For this review, take the finished solid that the model builds, in its own axes (mm). A direction names the side the tool comes from. Coordinates: 2 decimals unless noted, no trailing zeros. Write each loop counter-clockwise with the first axis right and the second up, starting at its lowest first coordinate (ties: lowest second). Pieces come first, ordered by that corner, then holes. Notation, with made-up numbers: M 66,6.5 L 121,6.5 A15 ccw 121,13.5 Z; hole C -36.75,25.5 d10. An arc over 180 degrees is marked long. Return JSON: item names as keys, results as strings.
```python
from build123d import *

# Parameters (mm, degrees)
ESQUISSE1_W             = 5
ESQUISSE1_H             = 83
BOSS_EXTRU_1_DEPTH      = 18
TROU_TARAUD_M4_D        = 3.3
ESQUISSE4_W             = 5
ESQUISSE4_H             = 63
ENL_V_MAT_EXTRU_1_DEPTH = 10


with BuildPart() as part:
    # Esquisse1 → Boss.-Extru.1 (new body)
    with BuildSketch(Plane.XY):
        with Locations((0, 36.5)):
            Rectangle(ESQUISSE1_W, ESQUISSE1_H)
    extrude(amount=-BOSS_EXTRU_1_DEPTH)

    # Trou taraudé M4 (through all)
    with Locations(Plane.XY):
        with Locations((0, 0), (0, 36.5), (0, 73)):
            Hole(TROU_TARAUD_M4_D / 2)

    # Esquisse4 → Enlèv. mat.-Extru.1 (cut)
    with BuildSketch(Plane.XY):
        with Locations((0, 36.5)):
            Rectangle(ESQUISSE4_W, ESQUISSE4_H)
    extrude(amount=-ENL_V_MAT_EXTRU_1_DEPTH, mode=Mode.SUBTRACT)


solid = part.part
```
1. Wall thickness on L1, parallel to Y at x = 0, z = -14.5; L2, parallel to Y at x = 0, z = -7.25; L3, parallel to X at y = 73, z = -3.5: over which ranges is each line inside the solid? List them lowest first. Write a range as from..to.
Checks:
{"L1": "-5..-1.65, 1.65..34.85, 38.15..71.35, 74.65..78", "L2": "-5..-1.65, 1.65..5, 68..71.35, 74.65..78", "L3": "-2.5..-1.65, 1.65..2.5"}
2. We need section A-A (y = 0). State the section outline as (x, z) points.
Checks:
{"outline": "M -2.5,-18 L -1.65,-18 L -1.65,0 L -2.5,0 Z; M 1.65,-18 L 2.5,-18 L 2.5,0 L 1.65,0 Z"}
3. For faces 1 (the face through (2, 37, -10)), 2 (the face through (0, -5, -9)), list the 3-axis set-ups (+Z, -Z, +X, -X, +Y, -Y) from which the entire face can be reached by the end or side of a thin tool; tool diameter is ignored.
Checks:
{"face 1": "+Z, +X, -X", "face 2": "+Z, -Z, +X, -X, -Y"}
4. We need section D-D (y = 36.5). State the section outline as (x, z) points, plus the area to 3 significant figures.
Checks:
{"outline": "M -2.5,-18 L -1.65,-18 L -1.65,-10 L -2.5,-10 Z; M 1.65,-18 L 2.5,-18 L 2.5,-10 L 1.65,-10 Z", "area": "13.6 mm2"}
5. We need section C-C (z = -16). State the section outline as (x, y) points, plus the area to 3 significant figures.
Checks:
{"outline": "M -2.5,-5 L 2.5,-5 L 2.5,78 L -2.5,78 Z; hole C 0,0 d3.3; hole C 0,36.5 d3.3; hole C 0,73 d3.3", "area": "389 mm2"}
6. We need section B-B (x = 0). State the section outline as (y, z) points, plus the area to 3 significant figures.
Checks:
{"outline": "M -5,-18 L -1.65,-18 L -1.65,0 L -5,0 Z; M 1.65,-18 L 34.85,-18 L 34.85,-10 L 5,-10 L 5,0 L 1.65,0 Z; M 38.15,-18 L 71.35,-18 L 71.35,0 L 68,0 L 68,-10 L 38.15,-10 Z; M 74.65,-18 L 78,-18 L 78,0 L 74.65,0 Z", "area": "719 mm2"}
